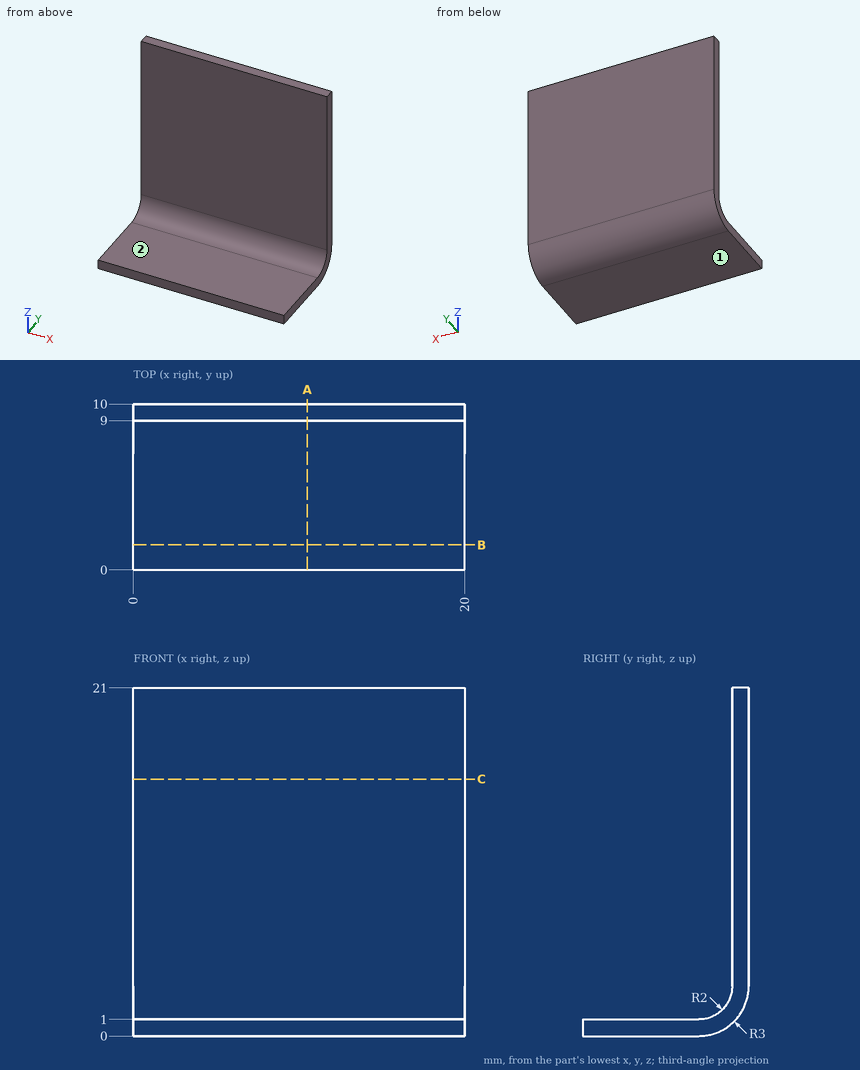
Here's the drawing with two shaded views (mm, measured from the low corner). I have some questions. A direction names the side the tool comes from. Give positions to 0.01 mm unless a question says otherwise; leave off trailing zeros. Order: outer loops, then holes, each group sorted by start corner. A loop starts at its lowest first (then second) coordinate and runs counter-clockwise, first axis right, second up.
Q1. I'm going to push flat-ended pins straight in: P1, Ø5.5, axis at x = 13.5, z = 10, coming from the -Y side; P2, Ø3, axis at x = 14, y = 3, coming from the +Z side; P3, Ø10, axis at x = 10.5, z = 7, coming from the -Y side. Where does each tip first touch, or does it pass through?
Q2. For the marked faces 1 and 2, which set-ups out of +Z, -Z, +X, -X, +Y, -Y let a thin tool reach every point of the face, with its end or its side?
Q3. Suppose I cut it at A-A, the plane x = 10.5. Write out the boundary of the cut face in (y, z).
Q4. Suppose I cut it at B-B, the plane y = 1.5. Write out the boundary of the cut face in (x, z), and give its area (3 significant figures).
Q5. Suppose I cut it at C-C, the plane z = 15.5. Write out the boundary of the cut face in (x, y), and give its area (3 significant figures).
Q6. If I drill on line 1 along Z through (x, y) = (16.25, 4.75); line 2 along Y through (x, z) = (10, 7.25); line 3 along Z through (x, y) = (16.75, 8.75), over which ranges is the centre line in solid material (lowest first)?
Solution:
1. P1: stops at y = 9
1. P2: stops at z = 1
1. P3: stops at y = 8.73
2. face 1: -Z, +X, -X, +Y, -Y
2. face 2: +Z, +X, -X, -Y
3. outline: (0, 0) - (7, 0) arc R3 ccw to (10, 3) - (10, 21) - (9, 21) - (9, 3) arc R2 cw to (7, 1) - (0, 1) - close
4. outline: (0, 0) - (20, 0) - (20, 1) - (0, 1) - close
4. area: 20.0 mm2
5. outline: (0, 9) - (20, 9) - (20, 10) - (0, 10) - close
5. area: 20.0 mm2
6. line 1: z = 0 to 1
6. line 2: y = 9 to 10
6. line 3: z = 0.56 to 2.03
